```python
from build123d import *

# Parameters (mm, degrees)
SKETCH1_R           = 7.5
SKETCH1_R_2         = 3.25
BOSS_EXTRUDE1_DEPTH = 15
FILLET1_R           = 20
FILLET2_R           = 20
FILLET3_R           = 20
FILLET4_R           = 20


with BuildPart() as part:
    # Sketch1 → Boss-Extrude1 (new body)
    with BuildSketch(Plane.XY):
        with BuildLine():
            Line((75, 50), (105, 50))
            Line((105, 50), (350, 50))
            Line((350, 50), (350, 3.7471e-05))
            Line((350, 3.7471e-05), (252.995324667, -19.768817559))
            ThreePointArc((252.995324667, -19.768817559), (250.90496409, -20.043601976), (248.796724988, -20.022585277))
            Line((248.796724988, -20.022585277), (0, 0))
            Line((0, 0), (0, 50))
            Line((0, 50), (75, 50))
        make_face()
        with Locations((25, 25)):
            Circle(SKETCH1_R, mode=Mode.SUBTRACT)
        with Locations((250, -5.070925528)):
            Circle(SKETCH1_R_2, mode=Mode.SUBTRACT)
    extrude(amount=BOSS_EXTRUDE1_DEPTH)

    # Fillet1
    fillet1_edges = [part.edges().sort_by_distance(p)[0] for p in [
        (0, 50, 7.5),
    ]]
    fillet(fillet1_edges, radius=FILLET1_R)

    # Fillet2
    fillet2_edges = [part.edges().sort_by_distance(p)[0] for p in [
        (0, 0, 7.5),
    ]]
    fillet(fillet2_edges, radius=FILLET2_R)

    # Fillet3
    fillet3_edges = [part.edges().sort_by_distance(p)[0] for p in [
        (350, 50, 7.5),
    ]]
    fillet(fillet3_edges, radius=FILLET3_R)

    # Fillet4
    fillet4_edges = [part.edges().sort_by_distance(p)[0] for p in [
        (350, 3.7471e-05, 7.5),
    ]]
    fillet(fillet4_edges, radius=FILLET4_R)


solid = part.part
```
Design review of the part built by this model. Coordinates are the model's own, in mm. Give positions to 0.01 mm unless a question says otherwise; leave off trailing zeros. Write each loop counter-clockwise with the first axis right and the second up, starting at its lowest first coordinate (ties: lowest second). Pieces come first, ordered by that corner, then holes. Notation, with made-up numbers: (16, 84.25) - (53, 84.25) arc R16 ccw to (53, 108.25) - close; hole circle Ø5 at (65, -32). An arc over 180 degrees is marked (long way). Return JSON: item names as keys, results as strings. Group by question number.
(1) We need section D-D, the plane x = 140.5. Give the boundary of the cut face in (y, z), then the cut area to 3 significant figures.
(2) We need section B-B, the plane z = 9.5. Give the boundary of the cut face in (x, y), then the cut area to 3 significant figures.
(3) We need section A-A, the plane y = 25. Give the boundary of the cut face in (x, z), then the cut area to 4 significant figures.
(4) Mouldability with a two-part tool opening along Y and no side actions: class faces 1 (the cylindrical face through (19.5, 30.1, 7.4)), 2 (the flat face through (0, 24, 7)), 3 (the cylindrical face through (246.753, -4.928, 7.395)), 4 (the cylindrical face through (345.61, 3.83, 7.6)) as +Y half, -Y half, draft (parallel to the pull), parting line (faces both ways), or undercut.
(5) To check wall thickness, follow probe 1 along Y at (x, z) = (250, 5.25); probe 2 along X at (y, z) = (27.5, 13.25); probe 3 along X at (y, z) = (25.5, 2.25). State the ranges of each line that lie inside material, in increasing order.
(6) We need section C-C, the plane x = 25. Give the boundary of the cut face in (y, z), then the cut area to 3 significant figures.
(7) Insertion check: pin 1 (4 mm diameter, centred on x = 67.5, z = 8, fed in from -Y); pin 2 (1 mm diameter, centred on x = 203.5, z = 6.5, fed in from -Y). Each pin has a flat end and moves straight along its axis. Give the tip position at first contact, or say it passes through.
Reported:
{
 "1": {"outline": "(-11.31, 0) - (50, 0) - (50, 15) - (-11.31, 15) - close", "area": "920 mm2"},
 "2": {"outline": "(0, 18.46) arc R20 ccw to (18.4, -1.48) - (248.8, -20.02) arc R15 ccw to (253, -19.77) - (333.99, -3.26) arc R20 ccw to (350, 16.34) - (350, 30) arc R20 ccw to (330, 50) - (20, 50) arc R20 ccw to (0, 30) - close; hole circle Ø15 at (25, 25); hole circle Ø6.5 at (250, -5.07)", "area": "20,500 mm2"},
 "3": {"outline": "(0, 0) - (17.5, 0) - (17.5, 15) - (0, 15) - close; (32.5, 0) - (350, 0) - (350, 15) - (32.5, 15) - close", "area": "5,025 mm2"},
 "4": {"face 1": "undercut", "face 2": "draft", "face 3": "undercut", "face 4": "-Y half"},
 "5": {"probe 1": "y = -20.07 to -8.32, -1.82 to 50", "probe 2": "x = 0 to 17.93, 32.07 to 350", "probe 3": "x = 0 to 17.52, 32.48 to 350"},
 "6": {"outline": "(-2.01, 0) - (17.5, 0) - (17.5, 15) - (-2.01, 15) - close; (32.5, 0) - (50, 0) - (50, 15) - (32.5, 15) - close", "area": "555 mm2"},
 "7": {"pin 1": "stops at y = -5.59", "pin 2": "stops at y = -16.42"}
}
